Could you check a few things on this model? Use its own coordinates, in mm. Round coordinates to 2 decimals unless told otherwise and drop trailing zeros. Loops run counter-clockwise (first coordinate to the right, second up) from the corner with the lowest first, then second, coordinate; pieces in that order, holes last. Notation, with made-up numbers: (-23.5, -5) - (23.5, -5) arc R21 cw to (23.5, 25) - close; hole circle Ø8 at (52, 58.25). An arc over 180 degrees is marked (long way). Answer as CSV lines item,"result". Start each with the question number.
1) Suppose I cut it at A-A, the plane y = -12.7. Write out the boundary of the cut face in (x, z) (3 decimals), then the cut area to 3 significant figures.
2) Suppose I cut it at D-D, the plane y = 21. Write out the boundary of the cut face in (x, z), then the cut area to 3 significant figures.
3) Suppose I cut it at C-C, the plane y = 13.5. Write out the boundary of the cut face in (x, z) (3 decimals).
4) Please list where these lines run through material, in increasing order: line 1 along X through (y, z) = (-12.5, 0.75) (3 decimals); line 2 along Y through (x, z) = (-26, 0.5); line 3 along Y through (x, z) = (0.5, 4.5).
5) We'd pull the mould along Y, two halves only. Please class faces 1 (the face through (0, 25.4, 3)), 2 (the face through (0, -25.4, 3)), 3 (the face through (-1, 0, 0)), 4 (the face through (22.86, 15.02, 3.13)): pulls with the +Y half, pulls with the -Y half, needs draft (parallel to the pull), parting line crosses it, or undercut.
6) I'm going to push flat-ended pins straight in: pin 1 Ø4.5 at (x, y) = (24.335, -12.7) entering from -Z; pin 2 Ø6.5 at (x, y) = (-26.465, -12.7) entering from +Z. Where does each tip first touch, or does it pass through?
7) Suppose I cut it at B-B, the plane z = 1.75. Write out the boundary of the cut face in (x, y) (3 decimals), then the cut area to 3 significant figures.
```python
from build123d import *

# Parameters (mm, degrees)
SKETCH1_W            = 74.07
SKETCH1_H            = 50.8
BOSS_EXTRUDE1_DEPTH  = 6.35
FILLET1_R            = 10
M5_CLEARANCE_HOLE1_D = 5.5


with BuildPart() as part:
    # Sketch1 → Boss-Extrude1 (new body)
    with BuildSketch(Plane.XY):
        Rectangle(SKETCH1_W, SKETCH1_H)
    extrude(amount=BOSS_EXTRUDE1_DEPTH)

    # Fillet1
    fillet1_edges = [part.edges().sort_by_distance(p)[0] for p in [
        (-37.035, 25.4, 3.175),
        (37.035, 25.4, 3.175),
        (37.035, -25.4, 3.175),
        (-37.035, -25.4, 3.175),
    ]]
    fillet(fillet1_edges, radius=FILLET1_R)

    # M5 Clearance Hole1 (through all)
    with Locations(Plane.XY.offset(6.35)):
        with Locations((-26.465, 12.7), (-26.465, -12.7), (-1.065, -12.7), (-1.065, 12.7), (24.335, 12.7), (24.335, -12.7)):
            Hole(M5_CLEARANCE_HOLE1_D / 2)


solid = part.part
```
Filled sheet:
1,outline,"(-37.035, 0) - (-29.215, 0) - (-29.215, 6.35) - (-37.035, 6.35) - close; (-23.715, 0) - (-3.815, 0) - (-3.815, 6.35) - (-23.715, 6.35) - close; (1.685, 0) - (21.585, 0) - (21.585, 6.35) - (1.685, 6.35) - close; (27.085, 0) - (37.035, 0) - (37.035, 6.35) - (27.085, 6.35) - close"
1,area,"366 mm²"
2,outline,"(-35.32, 0) - (35.32, 0) - (35.32, 6.35) - (-35.32, 6.35) - close"
2,area,"449 mm²"
3,outline,"(-37.035, 0) - (-29.096, 0) - (-29.096, 6.35) - (-37.035, 6.35) - close; (-23.834, 0) - (-3.696, 0) - (-3.696, 6.35) - (-23.834, 6.35) - close; (1.566, 0) - (21.704, 0) - (21.704, 6.35) - (1.566, 6.35) - close; (26.966, 0) - (37.035, 0) - (37.035, 6.35) - (26.966, 6.35) - close"
4,line 1,"-37.035 to -29.208, -23.722 to -3.808, 1.678 to 21.592, 27.078 to 37.035"
4,line 2,"-25.4 to -15.41, -9.99 to 9.99, 15.41 to 25.4"
4,line 3,"-25.4 to -14.96, -10.44 to 10.44, 14.96 to 25.4"
5,face 1,"pulls with the +Y half"
5,face 2,"pulls with the -Y half"
5,face 3,"needs draft"
5,face 4,"undercut"
6,pin 1,"through"
6,pin 2,"z = 6.35"
7,outline,"(-37.035, -15.4) arc R10 ccw to (-27.035, -25.4) - (27.035, -25.4) arc R10 ccw to (37.035, -15.4) - (37.035, 15.4) arc R10 ccw to (27.035, 25.4) - (-27.035, 25.4) arc R10 ccw to (-37.035, 15.4) - close; hole circle Ø5.5 at (-26.465, -12.7); hole circle Ø5.5 at (-26.465, 12.7); hole circle Ø5.5 at (-1.065, -12.7); hole circle Ø5.5 at (-1.065, 12.7); hole circle Ø5.5 at (24.335, -12.7); hole circle Ø5.5 at (24.335, 12.7)"
7,area,"3,530 mm²"
